The figure shows three views and two pictorial views of one solid part (mm, origin at its lowest corner). Answer the questions. Give positions to 0.01 mm unless a question says otherwise; leave off trailing zeros. Order: outer loops, then holes, each group sorted by start corner. A loop starts at its lowest first (then second) coordinate and runs counter-clockwise, first axis right, second up. Notation, with made-up numbers: (56.5, 15) - (81.5, 15) arc R24 cw to (81.5, 41) - close; hole circle Ø5 at (71, 24). An arc over 180 degrees is marked (long way). Answer as a JSON object with one key per item and string values. Group by question number.
Q1. Given pin 1 (5 mm diameter, centred on x = 22.5, z = 25.5, fed in from +Y); pin 2 (4.5 mm diameter, centred on x = 23, y = 33, fed in from +Z); pin 3 (12 mm diameter, centred on y = 26, z = 60, fed in from -X); pin 4 (9.5 mm diameter, centred on x = 20, z = 40, fed in from +Y), each flat-ended and moving along its own axis, determine where each tip first touches the part or whether it passes through.
Q2. A cutting plane is placed at B-B, the plane z = 16.5. Give the vertices of the cut face in (x, y).
Q3. Consider line 1 (Z direction, x = 20, y = 17); line 2 (Z direction, x = 15, y = 36); line 3 (Y direction, x = 8.5, z = 32). Determine where each line is inside the solid, lowest interval first.
Q4. A cutting plane is placed at D-D, the plane y = 35.5. Give the vertices of the cut face in (x, z), and give its area (3 significant figures).
Q5. A cutting plane is placed at C-C, the plane x = 35.5. Give the vertices of the cut face in (y, z).
Q6. A cutting plane is placed at A-A, the plane z = 40. Give the vertices of the cut face in (x, y), and give its area (3 significant figures).
Q7. The mould has two halves that part along Z. Classify the marked faces 1, 2, 3 and 4: released by +Z, released by -Z, zero draft, split by the parting line, or undercut.
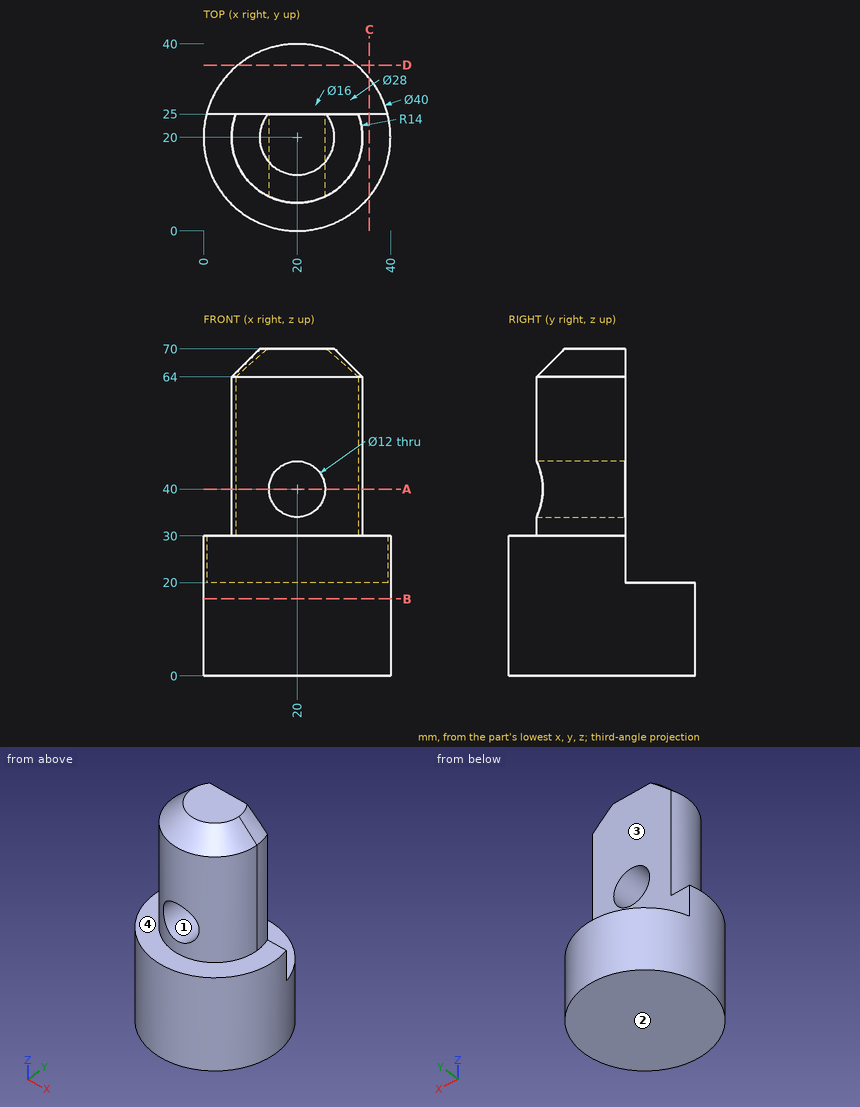
Reply:
{
 "1": {"pin 1": "stops at y = 25", "pin 2": "stops at z = 20", "pin 3": "stops at x = 6", "pin 4": "passes through"},
 "2": {"outline": "circle Ø40 at (20, 20)"},
 "3": {"line 1": "z = 0 to 34, 46 to 70", "line 2": "z = 0 to 20", "line 3": "y = 12.02 to 25"},
 "4": {"outline": "(7.36, 0) - (32.64, 0) - (32.64, 20) - (7.36, 20) - close", "area": "506 mm^2"},
 "5": {"outline": "(7.36, 0) - (32.64, 0) - (32.64, 20) - (25, 20) - (25, 30) - (7.36, 30) - close"},
 "6": {"outline": "(6.92, 25) arc R14 ccw to (14, 7.35) - (14, 25) - close; (26, 7.35) arc R14 ccw to (33.08, 25) - (26, 25) - close", "area": "222 mm^2"},
 "7": {"face 1": "undercut", "face 2": "released by -Z", "face 3": "zero draft", "face 4": "released by +Z"}
}
